Can you work these out from the drawing? Everything is in mm from the part's minimum corner. Round coordinates to 2 decimals unless told otherwise and drop trailing zeros. Order: outer loops, then holes, each group sorted by start corner. A loop starts at its lowest first (then second) coordinate and runs counter-clockwise, first axis right, second up. Notation, with made-up numbers: M 52,62 L 58,62 A15 cw 58,84 Z; hole C -21.5,-35.75 d3. An arc over 180 degrees is marked long. Write each question's results on one line, items separated by ' | '. Start each with the question number.
1. Suppose I cut it at D-D on z = 12. Write out the boundary of the cut face in (x, y), and give its area (3 significant figures).
2. Suppose I cut it at B-B on z = 90. Write out the boundary of the cut face in (x, y), and give its area (3 significant figures).
3. Suppose I cut it at C-C on y = 1.6. Write out the boundary of the cut face in (x, z), and give its area (3 significant figures).
4. Please list where these lines run through material, in increasing order: L1, parallel to Z at x = 40, y = 1.35; L2, parallel to Z at x = 38, y = 1.1; L3, parallel to X at y = 1.55, z = 87.5.
5. Suppose I cut it at A-A on x = 40. Write out the boundary of the cut face in (y, z), and give its area (3 significant figures).
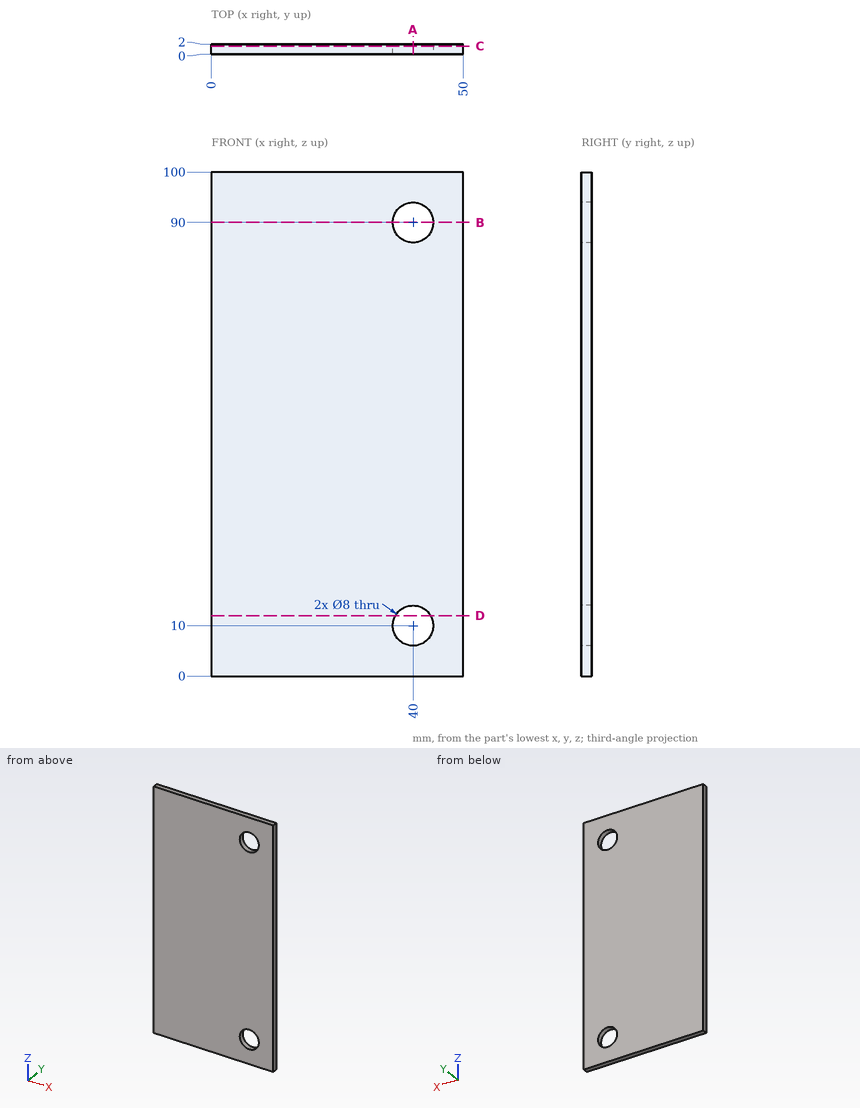
Filled sheet:
1) outline: M 0,0 L 36.54,0 L 36.54,2 L 0,2 Z; M 43.46,0 L 50,0 L 50,2 L 43.46,2 Z | area: 86.1 mm^2
2) outline: M 0,0 L 36,0 L 36,2 L 0,2 Z; M 44,0 L 50,0 L 50,2 L 44,2 Z | area: 84.0 mm^2
3) outline: M 0,0 L 50,0 L 50,100 L 0,100 Z; hole C 40,10 d8; hole C 40,90 d8 | area: 4,900 mm^2
4) L1: z = 0 to 6, 14 to 86, 94 to 100 | L2: z = 0 to 6.54, 13.46 to 86.54, 93.46 to 100 | L3: x = 0 to 36.88, 43.12 to 50
5) outline: M 0,0 L 2,0 L 2,6 L 0,6 Z; M 0,14 L 2,14 L 2,86 L 0,86 Z; M 0,94 L 2,94 L 2,100 L 0,100 Z | area: 168 mm^2
